Here's how the part is built. I have some questions about the finished solid (model axes, mm). Face numbers are marked on the shaded views. A direction names the side the tool comes from. Round coordinates to 2 decimals unless told otherwise and drop trailing zeros. Write each loop counter-clockwise with the first axis right and the second up, starting at its lowest first coordinate (ties: lowest second). Pieces come first, ordered by that corner, then holes. Notation, with made-up numbers: (42.25, -13.75) -> (83.25, -13.75) arc R8 ccw to (83.25, -7.75) -> close; hole circle Ø8 at (37, 61). An arc over 180 degrees is marked (long way). Answer as CSV lines item,"result".
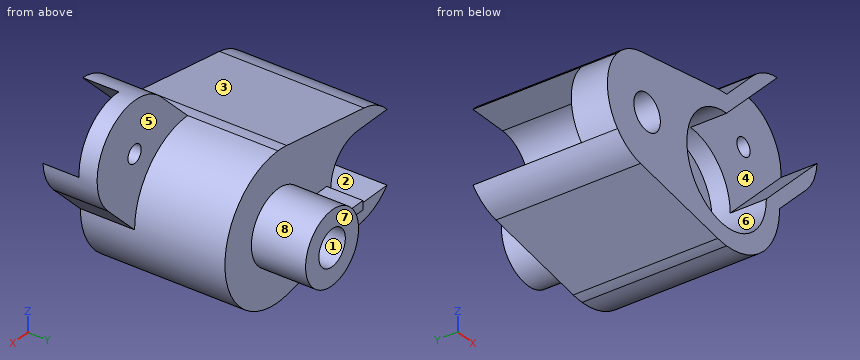
```python
from build123d import *

# Parameters (mm, degrees)
BOSS_EXTRUDE1_DEPTH        = 80
SKETCH2_R                  = 30
CUT_EXTRUDE1_DEPTH         = 30
SKETCH3_R                  = 20
BOSS_EXTRUDE2_DEPTH        = 30
F_20_0MM_DOWEL_HOLE1_D     = 20
F_20_0MM_DOWEL_HOLE1_DEPTH = 30
F_20_0MM_DOWEL_HOLE1_TIP   = 6.00860619
SKETCH6_R                  = 10
CUT_EXTRUDE2_DEPTH         = 109
SKETCH7_R                  = 10
CUT_EXTRUDE3_DEPTH         = 60
BOSS_EXTRUDE3_DEPTH        = 30
SKETCH11_R                 = 5
CUT_EXTRUDE4_DEPTH         = 30
SKETCH13_R                 = 5
CUT_EXTRUDE5_DEPTH         = 20
SKETCH14_W                 = 17
SKETCH14_H                 = 5
BOSS_EXTRUDE4_DEPTH        = 20


with BuildPart() as part:
    # Sketch1 → Boss-Extrude1 (new body)
    with BuildSketch(Plane(origin=(0, 0, 0), x_dir=(1, 0, 0), z_dir=(0, 1, 0))):
        with BuildLine():
            Line((-6.666666667, 39.440531887), (-65, 29.580398915))
            ThreePointArc((-65, 29.580398915), (-74.494747679, 26.265991124), (-82.360679775, 20))
            ThreePointArc((-82.360679775, 20), (-90, 0), (-82.360679775, -20))
            ThreePointArc((-82.360679775, -20), (-74.494747679, -26.265991124), (-65, -29.580398915))
            Line((-65, -29.580398915), (-6.666666667, -39.440531887))
            ThreePointArc((-6.666666667, -39.440531887), (-3.345050411, -39.859887578), (0, -40))
            ThreePointArc((0, -40), (40, 0), (0, 40))
            ThreePointArc((0, 40), (-3.345050411, 39.859887578), (-6.666666667, 39.440531887))
        make_face()
    extrude(amount=BOSS_EXTRUDE1_DEPTH)

    # Sketch2 → Cut-Extrude1 (cut)
    with BuildSketch(Plane.XZ):
        Circle(SKETCH2_R)
    extrude(amount=-CUT_EXTRUDE1_DEPTH, mode=Mode.SUBTRACT)

    # Sketch3 → Boss-Extrude2 (add)
    with BuildSketch(Plane(origin=(0, 80, 0), x_dir=(1, 0, 0), z_dir=(0, 1, 0))):
        Circle(SKETCH3_R)
    extrude(amount=BOSS_EXTRUDE2_DEPTH)

    # Ø20.0mm Dowel Hole1
    with Locations(Plane.ZX.offset(110)):
        with Locations((0, 0)):
            Hole(F_20_0MM_DOWEL_HOLE1_D / 2, depth=F_20_0MM_DOWEL_HOLE1_DEPTH)
            with Locations((0, 0, -(F_20_0MM_DOWEL_HOLE1_DEPTH + F_20_0MM_DOWEL_HOLE1_TIP / 2))):  # 118° drill point
                Cone(0, F_20_0MM_DOWEL_HOLE1_D / 2, F_20_0MM_DOWEL_HOLE1_TIP, mode=Mode.SUBTRACT)

    # Sketch6 → Cut-Extrude2 (cut)
    with BuildSketch(Plane(origin=(0, 80, 0), x_dir=(1, 0, 0), z_dir=(0, 1, 0))):
        with Locations((-60, 0)):
            Circle(SKETCH6_R)
    extrude(amount=-CUT_EXTRUDE2_DEPTH, mode=Mode.SUBTRACT)

    # Sketch7 → Cut-Extrude3 (cut)
    with BuildSketch(Plane(origin=(0, 80, 0), x_dir=(1, 0, 0), z_dir=(0, 1, 0))):
        with BuildLine():
            ThreePointArc((-60, -20), (-40, 0), (-60, 20))
            Line((-60, 20), (-82.360679775, 20))
            ThreePointArc((-82.360679775, 20), (-90, 0), (-82.360679775, -20))
            Line((-82.360679775, -20), (-60, -20))
        make_face()
        with Locations((-60, 0)):
            Circle(SKETCH7_R, mode=Mode.SUBTRACT)
    extrude(amount=-CUT_EXTRUDE3_DEPTH, mode=Mode.SUBTRACT)

    # Sketch10 → Boss-Extrude3 (add)
    with BuildSketch(Plane.XZ):
        with BuildLine():
            Line((20, 60), (0, 40))
            ThreePointArc((0, 40), (28.284271247, 28.284271247), (40, 0))
            Line((40, 0), (60, 20))
            ThreePointArc((60, 20), (60, 60), (20, 60))
        make_face()
    extrude(amount=-BOSS_EXTRUDE3_DEPTH)

    # Sketch11 → Cut-Extrude4 (cut)
    with BuildSketch(Plane(origin=(0, 0, 0), x_dir=(-1, 0, 0), z_dir=(0, -1, 0))):
        with Locations((-40, -40)):
            Circle(SKETCH11_R)
    extrude(amount=-CUT_EXTRUDE4_DEPTH, mode=Mode.SUBTRACT)

    # Sketch13 → Cut-Extrude5 (cut)
    with BuildSketch(Plane(origin=(0, 0, 0), x_dir=(-1, 0, 0), z_dir=(0, -1, 0))):
        with BuildLine():
            ThreePointArc((-68.228756555, -38.228756555), (-60, -60), (-38.228756555, -68.228756555))
            Line((-38.228756555, -68.228756555), (0, -30))
            ThreePointArc((0, -30), (-21.213203436, -21.213203436), (-30, 0))
            Line((-30, 0), (-68.228756555, -38.228756555))
        make_face()
        with Locations((-40, -40)):
            Circle(SKETCH13_R, mode=Mode.SUBTRACT)
    extrude(amount=-CUT_EXTRUDE5_DEPTH, mode=Mode.SUBTRACT)

    # Sketch14 → Boss-Extrude4 (add)
    with BuildSketch(Plane(origin=(0, 80, 0), x_dir=(1, 0, 0), z_dir=(0, 1, 0))):
        with Locations((-28.343134833, 0)):
            Rectangle(SKETCH14_W, SKETCH14_H)
    extrude(amount=BOSS_EXTRUDE4_DEPTH)


solid = part.part
```
1. Suppose I cut it at D-D on z = 53.5. Please give me the cut outline in (x, y), and give its area (3 significant figures).
Numbers:
outline,"(13.5, 0) -> (23.5, 0) -> (23.5, 20) -> (64.85, 20) -> (64.85, 30) -> (13.5, 30) -> close"
area,"714 mm^2"
2. If I drill on line 1 (Z direction, x = 0, y = 99); line 2 (X direction, y = 97, z = 0); line 3 (Y direction, x = 21.5, z = 54.5), over which ranges is the centre line in solid material (lowest first)?
Numbers:
line 1,"z = -20 to -10, 10 to 20"
line 2,"x = -36.84 to -10, 10 to 20"
line 3,"y = 0 to 30"
3. Suppose I cut it at B-B on z = 16. Please give me the cut outline in (x, y), and give its area (3 significant figures).
Numbers:
outline,"(-85.38, 0) -> (-25.38, 0) -> (-25.38, 30) -> (25.38, 30) -> (25.38, 20) -> (46, 20) -> (46, 0) -> (56, 0) -> (56, 30) -> (36.66, 30) -> (36.66, 80) -> (12, 80) -> (12, 110) -> (-12, 110) -> (-12, 80) -> (-48, 80) -> (-48, 20) -> (-85.38, 20) -> close"
area,"6,890 mm^2"
4. Suppose I cut it at C-C on z = -12. Please give me the cut outline in (x, y), and give its area (3 significant figures).
Numbers:
outline,"(-87.5, 0) -> (-27.5, 0) -> (-27.5, 30) -> (27.5, 30) -> (27.5, 0) -> (38.16, 0) -> (38.16, 80) -> (16, 80) -> (16, 110) -> (-16, 110) -> (-16, 80) -> (-44, 80) -> (-44, 20) -> (-87.5, 20) -> close"
area,"6,750 mm^2"
5. If we mould it in two halves opening along Z, with no side actions, what happens to the marked faces 6, 7 and 8? For each: released by +Z, released by -Z, zero draft, split by the parting line, or undercut.
Numbers:
face 6,"undercut"
face 7,"zero draft"
face 8,"split by the parting line"
6. For pin 1 Ø5.5 at (y, z) = (90.5, -0.5) entering from -X; pin 2 Ø24.5 at (x, y) = (-66.5, 63) entering from -Z; pin 3 Ø2 at (x, y) = (-4, 14.5) entering from -Z, each with a flat end and sliding along its axis, tell me the tip position at first contact or that it passes through.
Numbers:
pin 1,"stops at x = -36.84"
pin 2,"stops at z = -31.4"
pin 3,"stops at z = -39.89"
7. Suppose I cut it at A-A on y = 98. Please give me the cut outline in (x, z).
Numbers:
outline,"(-36.84, -2.5) -> (-19.84, -2.5) arc R20 ccw (long way) to (-19.84, 2.5) -> (-36.84, 2.5) -> close; hole circle Ø20 at (0, 0)"
8. On a 3-axis mill with a long thin cutter (end or side, diameter ignored), from which of +Z, -Z, +X, -X, +Y, -Y can I reach the whole of each face in a straight line? I mean the marked faces 1, 2, 3, 4 and 5. Say none if no direction works.
Numbers:
face 1,"+Y"
face 2,"-X, +Y"
face 3,"+Z, -X, +Y, -Y"
face 4,"-Y"
face 5,"+Z, +X, +Y"
